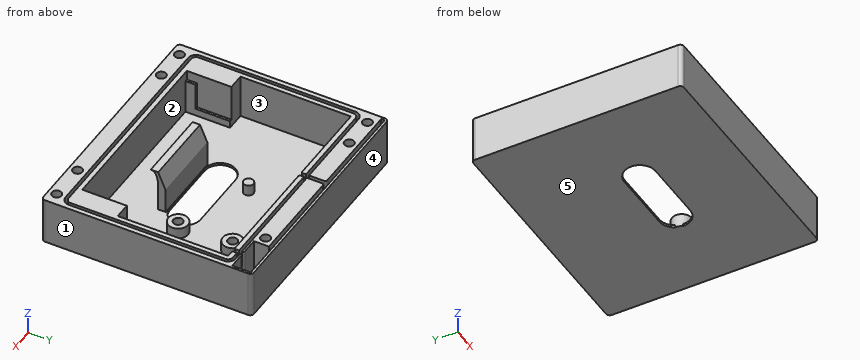
from build123d import *

# Parameters (mm, degrees)
PAD_DEPTH       = 1
PAD001_DEPTH    = 19
SKETCH002_R     = 4
SKETCH002_R_2   = 1.95
SKETCH002_R_3   = 2
PAD002_DEPTH    = 5.5
PAD003_DEPTH    = 15
POCKET_DEPTH    = 7
PAD004_DEPTH    = 1
SKETCH007_R     = 1.95
POCKET001_DEPTH = 5
PAD014_DEPTH    = 1


with BuildPart() as part:
    # Sketch → Pad (new body)
    with BuildSketch(Plane.XY):
        with BuildLine():
            Line((-47.5, -42.5), (47.5, -42.5))
            ThreePointArc((47.5, -42.5), (48.56066, -42.06066), (49, -41))
            Line((49, -41), (49, 41))
            ThreePointArc((49, 41), (48.56066, 42.06066), (47.5, 42.5))
            Line((47.5, 42.5), (-47.5, 42.5))
            ThreePointArc((-47.5, 42.5), (-48.56066, 42.06066), (-49, 41))
            Line((-49, 41), (-49, -41))
            ThreePointArc((-49, -41), (-48.56066, -42.06066), (-47.5, -42.5))
        make_face()
        with BuildLine():
            ThreePointArc((-12.5, 1.25), (-18.75, -5), (-12.5, -11.25))
            Line((-12.5, -11.25), (12.5, -11.25))
            ThreePointArc((12.5, -11.25), (18.75, -5), (12.5, 1.25))
            Line((-12.5, 1.25), (12.5, 1.25))
        make_face(mode=Mode.SUBTRACT)
    extrude(amount=PAD_DEPTH)

    # Sketch001 → Pad001 (join)
    with BuildSketch(Plane.XY):
        with BuildLine():
            Line((-47.5, -42.5), (47.5, -42.5))
            ThreePointArc((47.5, -42.5), (48.56066, -42.06066), (49, -41))
            Line((49, -41), (49, 41))
            ThreePointArc((49, 41), (48.56066, 42.06066), (47.5, 42.5))
            Line((47.5, 42.5), (-47.5, 42.5))
            ThreePointArc((-47.5, 42.5), (-48.56066, 42.06066), (-49, 41))
            Line((-49, 41), (-49, -41))
            ThreePointArc((-49, -41), (-48.56066, -42.06066), (-47.5, -42.5))
        make_face()
        with BuildLine():
            Line((44, 30.1), (44, -14.5))
            Line((44, -14.5), (37.5, -14.5))
            Line((37.5, -14.5), (37.5, -32.5))
            Line((37.5, -32.5), (-37.5, -32.5))
            Line((-37.5, -32.5), (-37.5, -14.5))
            Line((-37.5, -14.5), (-44, -14.5))
            Line((-44, -14.5), (-44, 30.1))
            Line((-44, 30.1), (-9.25, 30.1))
            ThreePointArc((-9.25, 30.1), (-8.71967, 30.31967), (-8.5, 30.85))
            Line((-8.5, 30.85), (-8.5, 39.35))
            ThreePointArc((-8.5, 39.35), (-8.71967, 39.88033), (-9.25, 40.1))
            Line((-9.25, 40.1), (-48, 40.1))
            Line((-48, 40.1), (-48, 41.5))
            Line((-48, 41.5), (48, 41.5))
            Line((48, 34), (48, 41.5))
            Line((48, 34), (41.5, 34))
            ThreePointArc((41.5, 34), (41.146447, 33.853553), (41, 33.5))
            Line((41, 33.5), (41, 30.6))
            ThreePointArc((41, 30.6), (41.146447, 30.246447), (41.5, 30.1))
            Line((41.5, 30.1), (44, 30.1))
        make_face(mode=Mode.SUBTRACT)
        with BuildLine():
            Line((-7, 30.85), (-7, 39.35))
            ThreePointArc((-6.25, 40.1), (-6.78033, 39.88033), (-7, 39.35))
            Line((-6.25, 40.1), (32.5, 40.1))
            Line((32.5, 40.1), (32.5, 34))
            Line((32.5, 34), (39, 34))
            ThreePointArc((39.5, 33.5), (39.353553, 33.853553), (39, 34))
            Line((39.5, 33.5), (39.5, 30.6))
            ThreePointArc((39, 30.1), (39.353553, 30.246447), (39.5, 30.6))
            Line((39, 30.1), (-6.25, 30.1))
            ThreePointArc((-7, 30.85), (-6.78033, 30.31967), (-6.25, 30.1))
        make_face()
    extrude(amount=PAD001_DEPTH)

    # Sketch002 → Pad002 (join)
    with BuildSketch(Plane.XY):
        with Locations((22, 19.5)):
            Circle(SKETCH002_R)
        with Locations((22, 19.5)):
            Circle(SKETCH002_R_2, mode=Mode.SUBTRACT)
        with Locations((22, -2.5)):
            Circle(SKETCH002_R)
        with Locations((22, -2.5)):
            Circle(SKETCH002_R_2, mode=Mode.SUBTRACT)
        with Locations((-9, 8.5)):
            Circle(SKETCH002_R_3)
    extrude(amount=PAD002_DEPTH)

    # Sketch003 → Pad003 (join, symmetric)
    with BuildSketch(Plane.YZ):
        with BuildLine():
            Line((-14.5, 0), (-14.5, 11))
            add(Edge.make_bspline(
                [(-17.5, 18), (-14.5, 18), (-14.5, 11)],
                knots=[0, 0, 0, 1, 1, 1], degree=2))
            Line((-17.5, 18), (-14.5, 18))
            Line((-14.5, 18), (-11.5, 11))
            Line((-11.5, 11), (-11.5, 0))
            Line((-11.5, 0), (-14.5, 0))
        make_face()
    extrude(amount=PAD003_DEPTH, both=True)

    # Sketch004 (on Face14 of Pad003) → Pocket (cut)
    with BuildSketch(Plane.XY.offset(19)):
        with BuildLine():
            Line((47.1, -32.5), (47.1, 30.1))
            ThreePointArc((47.1, 30.1), (46.192031, 32.292031), (44, 33.2))
            Line((44, 33.2), (-44, 33.2))
            ThreePointArc((-44, 33.2), (-46.192031, 32.292031), (-47.1, 30.1))
            Line((-47.1, 30.1), (-47.1, -32.5))
            ThreePointArc((-47.1, -32.5), (-46.192031, -34.692031), (-44, -35.6))
            Line((-44, -35.6), (44, -35.6))
            ThreePointArc((44, -35.6), (46.192031, -34.692031), (47.1, -32.5))
        make_face()
        with BuildLine():
            Line((45.9, -32.5), (45.9, 30.1))
            ThreePointArc((45.9, 30.1), (45.343503, 31.443503), (44, 32))
            Line((44, 32), (-44, 32))
            ThreePointArc((-44, 32), (-45.343503, 31.443503), (-45.9, 30.1))
            Line((-45.9, 30.1), (-45.9, -32.5))
            ThreePointArc((-45.9, -32.5), (-45.343503, -33.843503), (-44, -34.4))
            Line((-44, -34.4), (44, -34.4))
            ThreePointArc((44, -34.4), (45.343503, -33.843503), (45.9, -32.5))
        make_face(mode=Mode.SUBTRACT)
    extrude(amount=-POCKET_DEPTH, mode=Mode.SUBTRACT)

    # Sketch005 → Pad004 (join)
    with BuildSketch(Plane.YZ.offset(36.5)):
        Polygon((-14.5, 0), (-14.5, 4), (-28.5, 4), (-28.5, 15), (-32.5, 15), (-32.5, 0), align=None)
    extrude(amount=PAD004_DEPTH)

    # Sketch007 (on DatumPlane) → Pocket001 (cut)
    with BuildSketch(Plane.XY.offset(19)):
        with Locations((-44, -39.166667)):
            Circle(SKETCH007_R)
        with Locations((44, -39.166667)):
            Circle(SKETCH007_R)
        with Locations((-44, 36.766667)):
            Circle(SKETCH007_R)
        with Locations((29, 36.766667)):
            Circle(SKETCH007_R)
        with Locations((-31, 36.766667)):
            Circle(SKETCH007_R)
        with Locations((29, -39.166667)):
            Circle(SKETCH007_R)
        with Locations((-31, -39.166667)):
            Circle(SKETCH007_R)
    extrude(amount=-POCKET001_DEPTH, mode=Mode.SUBTRACT)

    # Sketch006 → Pad014 (join)
    with BuildSketch(Plane.YZ.offset(-37.5)):
        Polygon((-32.5, 0), (-32.5, 15), (-28.5, 15), (-28.5, 4), (-14.5, 4), (-14.5, 0), align=None)
    extrude(amount=PAD014_DEPTH)


solid = part.part
Work out the finished part from the listing and answer in its coordinate system (mm). Face numbers are marked on the shaded views. A direction names the side the tool comes from. Round coordinates to 2 decimals unless told otherwise and drop trailing zeros. Order: outer loops, then holes, each group sorted by start corner. A loop starts at its lowest first (then second) coordinate and runs counter-clockwise, first axis right, second up. Notation, with made-up numbers: M 78,-13 L 102,-13 A26 ccw 102,20 Z; hole C 36.5,11.25 d6. An arc over 180 degrees is marked long. One line per item, written item: value.
Q1. Find section B-B on x = -28. Write down the section's boundary in (y, z).
Derived:
outline: M -42.5,0 L 42.5,0 L 42.5,19 L 41.5,19 L 41.5,1 L 40.1,1 L 40.1,19 L 33.2,19 L 33.2,12 L 32,12 L 32,19 L 30.1,19 L 30.1,1 L -32.5,1 L -32.5,19 L -34.4,19 L -34.4,12 L -35.6,12 L -35.6,19 L -42.5,19 Z
Q2. Determine the mould class of the marked faces 3, 4 and 5 for opening direction Y: released by +Y, released by -Y, zero draft, split by the parting line, or undercut.
Derived:
face 3: undercut
face 4: released by +Y
face 5: zero draft
Q3. Flat-ended cylindrical pins translate along their axes: pin 1 (12 mm diameter, centred on x = -39, y = 10.5, fed in from +Z); pin 2 (1.9 mm diameter, centred on x = 29.5, y = 36, fed in from +Z); pin 3 (4 mm diameter, centred on x = -35, y = 18, fed in from +Z). Find the tip coordinate at first contact, or state that the pin passes through.
Derived:
pin 1: z = 19
pin 2: z = 14
pin 3: z = 1
Q4. Find section D-D on y = -30. Write down the section's boundary in (x, z), then the cut area to 3 significant figures.
Derived:
outline: M -49,0 L 49,0 L 49,19 L 47.1,19 L 47.1,12 L 45.9,12 L 45.9,19 L 37.5,19 L 37.5,15 L 36.5,15 L 36.5,1 L -36.5,1 L -36.5,15 L -37.5,15 L -37.5,19 L -45.9,19 L -45.9,12 L -47.1,12 L -47.1,19 L -49,19 Z
area: 523 mm²
Q5. Find section A-A on y = 19.5. Write down the section's boundary in (x, z), then the cut area to 3 significant figures.
Derived:
outline: M -49,0 L 49,0 L 49,19 L 47.1,19 L 47.1,12 L 45.9,12 L 45.9,19 L 44,19 L 44,1 L 26,1 L 26,5.5 L 23.95,5.5 L 23.95,1 L 20.05,1 L 20.05,5.5 L 18,5.5 L 18,1 L -44,1 L -44,19 L -45.9,19 L -45.9,12 L -47.1,12 L -47.1,19 L -49,19 Z
area: 280 mm²
Q6. For the marked faces 1 and 2, determine the directions among +Z, -Z, +X, -X, +Y, -Y from which every point of the face is accessible in a straight line to the end or side of a thin tool.
Derived:
face 1: +Z, -Z, +X, +Y, -Y
face 2: +Z
Q7. Find section C-C on z = 7.5. Give the number of separate pieces and of enclosed holes in the cut face, then the cut area to 3 significant figures.
Derived:
separate pieces: 3
enclosed holes: 1
area: 2,900 mm²
Q8. Straight lines are drawn through the part: line 1 (Y direction, x = 21, z = 16.25); line 2 (Y direction, x = -2, z = 5.5); line 3 (X direction, y = -25, z = 12.75). For each, find the intervals that lie inside material, in ascending order.
Derived:
line 1: -42.5 to -35.6, -34.4 to -32.5, 30.1 to 32, 33.2 to 40.1, 41.5 to 42.5
line 2: -42.5 to -32.5, -14.5 to -11.5, 30.1 to 40.1, 41.5 to 42.5
line 3: -49 to -47.1, -45.9 to -37.5, 37.5 to 45.9, 47.1 to 49
